Build history of the part. All positions in model axes, mm. A direction names the side the tool comes from. Give positions to 0.01 mm unless a question says otherwise; leave off trailing zeros. Write each loop counter-clockwise with the first axis right and the second up, starting at its lowest first coordinate (ties: lowest second). Pieces come first, ordered by that corner, then holes. Notation, with made-up numbers: (-32.5, 66.5) -> (10.5, 66.5) arc R20 cw to (10.5, 100.5) -> close; hole circle Ø9 at (66, -35.75). An arc over 180 degrees is marked (long way). One line per question, with ' | ' between items. Start each with the question number.
(1) Band-saw the part on C-C, the plane z = 72.5. Give the cut face in (x, y) (3 decimals), and give its area (3 significant figures).
(2) Band-saw the part on D-D, the plane x = -7. Give the cut face in (y, z).
(3) Drill centre lines: probe 1 along Z at (x, y) = (-3, -20.5); probe 2 along Y at (x, z) = (23.5, 18.5) (3 decimals); probe 3 along X at (y, z) = (-3, 61). Where is each one in solid material? Low to high. Write a range as from..to.
(4) Pin check, flat tips, straight feed: P1, Ø15.5, axis at x = -8, y = -6.5, coming from the -Z side; P2, Ø6, axis at x = -13.5, y = -22.5, coming from the +Z side. Stop position of each tip, or through.
(5) Band-saw the part on B-B, the plane y = 13. Give the cut face in (x, z).
(6) Band-saw the part on A-A, the plane x = -15. Give the cut face in (y, z), and give its area (3 significant figures).
(7) Pull direction Z, two halves, no side cores. Call faces 1 (the flat face through (-4, -4, 10)), 2 (the flat face through (-18.69, -10.16, 4.93)), 3 (the flat face through (-3, 3, 0)): released by +Z, released by -Z, zero draft, split by the parting line, or undercut.
(8) Tool access for faces 4 (the flat face through (-5, 2, 45)), 5 (the flat face through (11.77, -7.43, 34.37)): list every direction of +Z, -Z, +X, -X, +Y, -Y with a clear straight run to the whole face (end or side of a thin tool).
Autodesk Inventor part; units mm, degrees
ref_plane "YZ Plane" through (0, 0, 0) normal (1, 0, 0) x (0, 1, 0)
ref_plane "XZ Plane" through (0, 0, 0) normal (0, 1, 0) x (-1, 0, 0)
sketch "Эскиз1" plane through (0, 0, 0) normal (0, 0, 1) x (1, 0, 0)
  circle A0 centre (0, 0) radius 45
  line L0 (0, -45) -> (-38.9711, 22.5)
  line L1 (-38.9711, 22.5) -> (38.9711, 22.5)
  line L2 (38.9711, 22.5) -> (0, -45)
  dimension "d0" = 90
ref_plane "РабПлоскость1" through (0, 0, 90) normal (0, 0, 1) x (1, 0, 0)
sketch "Эскиз5" plane through (0, 0, 0) normal (0, 1, 0) x (-1, 0, 0)
  point P0 (0, 0)
sketch "Эскиз6" plane through (0, 0, 0) normal (1, 0, 0) x (0, 1, 0)
  point P0 (0, 0)
sketch "Эскиз7" plane through (0, 0, 0) normal (0, 1, 0) x (-1, 0, 0)
  point P0 (0, 0)
sketch "Эскиз8" plane through (0, 0, 90) normal (0, 0, 1) x (1, 0, 0)
  point P0 (0, 0)
loft "Лофт2" add profiles "Эскиз1" section 1 point at (0, 0, 90) contours L2 L0 L1
sketch "Эскиз9" plane through (0, 0, 0) normal (0, 1, 0) x (-1, 0, 0)
  point P0 (0, 0)
sketch "Эскиз10" plane through (0, 0, 0) normal (0, 1, 0) x (-1, 0, 0)
  line L0 (0, 10) -> (34.641, 10)
  line L1 (0, 90) -> (38.9711, 0)
  line L2 (0, 45) -> (19.4856, 45)
  line L3 (0, 45) -> (-15.1554, 10)
  line L4 (0, 90) -> (-38.9711, 0)
  line L5 (-15.1554, 10) -> (0, 10)
  line L6 (19.4856, 45) -> (34.641, 10)
  point P0 (0, 0)
extrude "Выдавливание1" cut sketch "Эскиз10" along normal mid plane 10000
properties part number "Деталь2Инди1"
Results:
1) outline: (-7.578, 4.375) -> (0, -8.75) -> (7.578, 4.375) -> close | area: 99.5 mm²
2) outline: (-32.88, 0) -> (22.5, 0) -> (20, 10) -> (-27.88, 10) -> close; (-10.38, 45) -> (11.25, 45) -> (4.04, 73.83) -> close
3) probe 1: z = 0..10 | probe 2: y = 4.953..17.875 | probe 3: x = -6.64..6.64
4) P1: stops at z = 0 | P2: stops at z = 10
5) outline: (-33.49, 0) -> (33.49, 0) -> (22.52, 38) -> (3.03, 38) -> (15.16, 10) -> (-30.6, 10) -> close
6) outline: (-19.02, 0) -> (22.5, 0) -> (20, 10) -> (-14.02, 10) -> close; (3.48, 45) -> (11.25, 45) -> (8.66, 55.36) -> close | area: 418 mm²
7) face 1: undercut | face 2: released by +Z | face 3: released by -Z
8) face 4: -X, +Y, -Y | face 5: +Z, +X, -Y
